Read the model definition and answer for the solid it produces. Units are mm, in the model's axes. A direction names the side the tool comes from. Give positions to 0.01 mm unless a question says otherwise; leave off trailing zeros. Order: outer loops, then holes, each group sorted by start corner. A loop starts at its lowest first (then second) coordinate and runs counter-clockwise, first axis right, second up. Notation, with made-up numbers: M 76,20 L 127,20 A22 ccw 127,36 Z; hole C 74.25,26 d5. An arc over 180 degrees is marked long. One line per item, written item: value.
from build123d import *

# Parameters (mm, degrees)
SKETCH2_W                       = 200
SKETCH2_H                       = 50
SKETCH2_R                       = 19
SKETCH2_R_2                     = 3.55
BOSS_EXTRUDE1_DEPTH             = 5
BOSS_EXTRUDE3_REACH             = 27
BOSS_EXTRUDE3_DIRECTION_2_REACH = 27
CUT_EXTRUDE2_DEPTH              = 20
CUT_EXTRUDE2_DEPTH_BACK         = 20
SKETCH8_R                       = 12.75
SKETCH8_R_2                     = 10.05
BOSS_EXTRUDE4_DEPTH             = 30.2
FILLET1_R                       = 5
SKETCH9_R                       = 3.5
CUT_EXTRUDE3_DEPTH              = 51
SKETCH13_R                      = 2
CUT_EXTRUDE5_DEPTH              = 2.5
CUT_EXTRUDE6_DEPTH              = 6
BOSS_EXTRUDE7_DEPTH             = 72
SKETCH17_R                      = 7.5
BOSS_EXTRUDE8_DEPTH             = 4
SKETCH18_R                      = 10.05
BOSS_EXTRUDE9_DEPTH             = 9.5
SKETCH19_W                      = 2.5
SKETCH19_H                      = 10
BOSS_EXTRUDE10_DEPTH            = 20
SKETCH20_R                      = 2.5
CUT_EXTRUDE7_DEPTH              = 36
SKETCH21_W                      = 3.5
SKETCH21_H                      = 5
CUT_EXTRUDE8_DEPTH              = 54.5


with BuildPart() as part:
    # Sketch2 → Boss-Extrude1 (new body)
    with BuildSketch(Plane(origin=(0, 0, 0), x_dir=(1, 0, 0), z_dir=(0, 1, 0))):
        Rectangle(SKETCH2_W, SKETCH2_H)
        with Locations((-60, 0)):
            Circle(SKETCH2_R, mode=Mode.SUBTRACT)
        with Locations((-31, 0)):
            Circle(SKETCH2_R_2, mode=Mode.SUBTRACT)
        with Locations((-89, 0)):
            Circle(SKETCH2_R_2, mode=Mode.SUBTRACT)
    extrude(amount=BOSS_EXTRUDE1_DEPTH)

    # Boss-Extrude3: up to this face of the body (flat: up to its plane)
    boss_extrude3_end = Plane(part.part.faces().sort_by_distance((0, 2.5, -25))[0])
    # Sketch6 → Boss-Extrude3 (add, up to the picked face)
    with BuildSketch(Plane.XY, mode=Mode.PRIVATE) as boss_extrude3_sk1:
        with BuildLine():
            Line((-100, 5), (-2.990738274, 34.75169137))
            ThreePointArc((-2.990738274, 34.75169137), (0, 35.2), (2.990738274, 34.75169137))
            Line((2.990738274, 34.75169137), (100, 5))
            Line((100, 5), (-100, 5))
        make_face()
    boss_extrude3_tool1 = split(extrude(boss_extrude3_sk1.sketch, amount=-BOSS_EXTRUDE3_REACH, mode=Mode.PRIVATE), bisect_by=boss_extrude3_end, keep=Keep.BOTH, mode=Mode.PRIVATE)
    add(boss_extrude3_tool1.solids().sort_by_distance((0, 15.216769, 0))[0])

    # Boss-Extrude3 direction 2: up to this face of the body (flat: up to its plane)
    boss_extrude3_direction_2_end = Plane(part.part.faces().sort_by_distance((0, 2.5, 25))[0])
    # Sketch6 → Boss-Extrude3 direction 2 (add, up to the picked face)
    with BuildSketch(Plane.XY, mode=Mode.PRIVATE) as boss_extrude3_direction_2_sk1:
        with BuildLine():
            Line((-100, 5), (-2.990738274, 34.75169137))
            ThreePointArc((-2.990738274, 34.75169137), (0, 35.2), (2.990738274, 34.75169137))
            Line((2.990738274, 34.75169137), (100, 5))
            Line((100, 5), (-100, 5))
        make_face()
    boss_extrude3_direction_2_tool1 = split(extrude(boss_extrude3_direction_2_sk1.sketch, amount=BOSS_EXTRUDE3_DIRECTION_2_REACH, mode=Mode.PRIVATE), bisect_by=boss_extrude3_direction_2_end, keep=Keep.BOTH, mode=Mode.PRIVATE)
    add(boss_extrude3_direction_2_tool1.solids().sort_by_distance((0, 15.216769, 0))[0])

    # Sketch7 → Cut-Extrude2 (cut, two sides)
    with BuildSketch(Plane.XY) as cut_extrude2_sk:
        with BuildLine():
            Line((2.990738274, 34.75169137), (100, 5))
            Line((100, 5), (-100, 5))
            Line((-100, 5), (-2.990738274, 34.75169137))
            ThreePointArc((-2.990738274, 34.75169137), (0, 35.2), (2.990738274, 34.75169137))
        make_face()
    extrude(amount=CUT_EXTRUDE2_DEPTH, mode=Mode.SUBTRACT)
    extrude(cut_extrude2_sk.sketch, amount=-CUT_EXTRUDE2_DEPTH_BACK, mode=Mode.SUBTRACT)

    # Sketch8 → Boss-Extrude4 (add)
    with BuildSketch(Plane(origin=(0, 5, 0), x_dir=(1, 0, 0), z_dir=(0, 1, 0))):
        Circle(SKETCH8_R)
        Circle(SKETCH8_R_2, mode=Mode.SUBTRACT)
    extrude(amount=BOSS_EXTRUDE4_DEPTH)

    # Fillet1
    fillet1_edges = [part.edges().sort_by_distance(p)[0] for p in [
        (0, 0, -25),
        (0, 0, 25),
    ]]
    fillet(fillet1_edges, radius=FILLET1_R)

    # Sketch9 → Cut-Extrude3 (cut, through all)
    with BuildSketch(Plane.XY.offset(25)):
        with Locations((0, 25)):
            Circle(SKETCH9_R)
    extrude(amount=-CUT_EXTRUDE3_DEPTH, mode=Mode.SUBTRACT)

    # Sketch13 → Cut-Extrude5 (cut)
    with BuildSketch(Plane(origin=(0, 5, 0), x_dir=(1, 0, 0), z_dir=(0, 1, 0))):
        with BuildLine():
            Line((23.5, 7.5), (53.5, 7.5))
            ThreePointArc((53.5, 7.5), (61, 0), (53.5, -7.5))
            Line((53.5, -7.5), (23.5, -7.5))
            ThreePointArc((23.5, -7.5), (16, 0), (23.5, 7.5))
        make_face()
        with Locations((31.5, 0)):
            Circle(SKETCH13_R, mode=Mode.SUBTRACT)
        with Locations((24.5, 0)):
            Circle(SKETCH13_R, mode=Mode.SUBTRACT)
        with Locations((38.5, 0)):
            Circle(SKETCH13_R, mode=Mode.SUBTRACT)
        with Locations((45.5, 0)):
            Circle(SKETCH13_R, mode=Mode.SUBTRACT)
        with Locations((52.5, 0)):
            Circle(SKETCH13_R, mode=Mode.SUBTRACT)
    extrude(amount=-CUT_EXTRUDE5_DEPTH, mode=Mode.SUBTRACT)

    # Sketch15 → Cut-Extrude6 (cut, through all)
    with BuildSketch(Plane(origin=(0, 5, 0), x_dir=(1, 0, 0), z_dir=(0, 1, 0))):
        with BuildLine():
            Line((23.5, 4), (53.5, 4))
            Line((53.5, 4), (100, 4))
            Line((100, 4), (100, -4))
            Line((100, -4), (53.5, -4))
            Line((53.5, -4), (23.5, -4))
            ThreePointArc((23.5, -4), (19.5, 0), (23.5, 4))
        make_face()
    extrude(amount=-CUT_EXTRUDE6_DEPTH, mode=Mode.SUBTRACT)

    # Sketch16 → Boss-Extrude7 (add)
    with BuildSketch(Plane(origin=(0, 5, 0), x_dir=(1, 0, 0), z_dir=(0, 1, 0))):
        with BuildLine():
            Line((16, -4), (16, -6.614378278))
            ThreePointArc((16, -6.614378278), (19.385621722, -9.114378278), (23.5, -10))
            Line((23.5, -10), (53.5, -10))
            Line((53.5, -10), (53.5, -7.5))
            Line((53.5, -7.5), (23.5, -7.5))
            ThreePointArc((23.5, -7.5), (19.877155813, -6.566962768), (17.15571123, -4))
            Line((17.15571123, -4), (16, -4))
        make_face()
        with BuildLine():
            Line((53.5, 10), (23.5, 10))
            ThreePointArc((23.5, 10), (19.385621722, 9.114378278), (16, 6.614378278))
            Line((16, 6.614378278), (16, 4))
            Line((16, 4), (17.15571123, 4))
            ThreePointArc((17.15571123, 4), (19.877155813, 6.566962768), (23.5, 7.5))
            Line((23.5, 7.5), (53.5, 7.5))
            Line((53.5, 7.5), (53.5, 10))
        make_face()
    extrude(amount=BOSS_EXTRUDE7_DEPTH)

    # Sketch17 → Boss-Extrude8 (add)
    with BuildSketch(Plane(origin=(0, 77, 0), x_dir=(1, 0, 0), z_dir=(0, 1, 0))):
        with BuildLine():
            Line((23.5, -10), (53.5, -10))
            Line((53.5, -10), (53.5, 10))
            Line((53.5, 10), (23.5, 10))
            ThreePointArc((23.5, 10), (19.385621722, 9.114378278), (16, 6.614378278))
            Line((16, 6.614378278), (16, 4))
            Line((16, 4), (16, -4))
            Line((16, -4), (16, -6.614378278))
            ThreePointArc((16, -6.614378278), (19.385621722, -9.114378278), (23.5, -10))
        make_face()
        with Locations((38.5, 0)):
            Circle(SKETCH17_R, mode=Mode.SUBTRACT)
    extrude(amount=BOSS_EXTRUDE8_DEPTH)

    # Sketch18 → Boss-Extrude9 (add)
    with BuildSketch(Plane(origin=(0, 5, 0), x_dir=(1, 0, 0), z_dir=(0, 1, 0))):
        Circle(SKETCH18_R)
    extrude(amount=BOSS_EXTRUDE9_DEPTH)

    # Sketch19 → Boss-Extrude10 (add)
    with BuildSketch(Plane(origin=(53.5, 0, 0), x_dir=(0, 0, -1), z_dir=(1, 0, 0))):
        with Locations((-8.75, 57)):
            Rectangle(SKETCH19_W, SKETCH19_H)
        with Locations((8.75, 57)):
            Rectangle(SKETCH19_W, SKETCH19_H)
        with Locations((8.75, 29)):
            Rectangle(SKETCH19_W, SKETCH19_H)
        with Locations((-8.75, 29)):
            Rectangle(SKETCH19_W, SKETCH19_H)
    extrude(amount=BOSS_EXTRUDE10_DEPTH)

    # Sketch20 → Cut-Extrude7 (cut, through all)
    with BuildSketch(Plane.XY.offset(10)):
        with Locations((66, 57)):
            Circle(SKETCH20_R)
        with Locations((66, 29)):
            Circle(SKETCH20_R)
    extrude(amount=-CUT_EXTRUDE7_DEPTH, mode=Mode.SUBTRACT)

    # Sketch21 → Cut-Extrude8 (cut)
    with BuildSketch(Plane(origin=(100, 0, 0), x_dir=(0, 0, -1), z_dir=(1, 0, 0))):
        with Locations((-5.75, 2.5)):
            Rectangle(SKETCH21_W, SKETCH21_H)
        with Locations((5.75, 2.5)):
            Rectangle(SKETCH21_W, SKETCH21_H)
    extrude(amount=-CUT_EXTRUDE8_DEPTH, mode=Mode.SUBTRACT)


solid = part.part
1) Consider probe 1 along Z at (x, y) = (36.5, 16); probe 2 along Y at (x, z) = (66, -8.2); probe 3 along Z at (x, y) = (-24.5, 6). Determine where each line is inside the solid, lowest interval first.
Reported:
probe 1: z = -25 to -20, -10 to -7.5, 7.5 to 10, 20 to 25
probe 2: y = 0 to 5, 24 to 26.5, 31.5 to 34, 52 to 54.5, 59.5 to 62
probe 3: z = -25 to -20, 20 to 25
2) Determine the mould class of faces 6 (the face through (1, 2, 24)), 7 (the face through (-1, 13, -25)), 8 (the face through (31, 2.5, 5)) for opening direction Y: +Y half, -Y half, draft (parallel to the pull), parting line (faces both ways), or undercut.
Reported:
face 6: -Y half
face 7: draft
face 8: undercut
3) Find section D-D, the plane x = 41. Write down the section's boundary in (y, z), plus the area to 3 significant figures.
Reported:
outline: M 0,-20 A5 ccw 5,-25 L 23.09,-25 L 23.09,-20 L 5,-20 L 5,-10 L 81,-10 L 81,-7.07 L 77,-7.07 L 77,-7.5 L 2.5,-7.5 L 2.5,-4 L 0,-4 Z; M 0,4 L 2.5,4 L 2.5,7.5 L 77,7.5 L 77,7.07 L 81,7.07 L 81,10 L 5,10 L 5,20 L 23.09,20 L 23.09,25 L 5,25 A5 ccw 0,20 Z
area: 746 mm^2
4) Find section C-C, the plane x = -56. Write down the section's boundary in (y, z).
Reported:
outline: M 0,-20 A5 ccw 5,-25 L 18.49,-25 L 18.49,-20 L 5,-20 L 5,-18.57 L 0,-18.57 Z; M 0,18.57 L 5,18.57 L 5,20 L 18.49,20 L 18.49,25 L 5,25 A5 ccw 0,20 Z
5) Which of the six approach directions +Z, -Z, +X, -X, +Y, -Y give full straight-line access (tool end or side, diameter ignored) to faces 1 (the face through (1, 14, -20)), 2 (the face through (43, 42, 10)), 3 (the face through (53.5, 78, 0)), 4 (the face through (45, 29, -7.5)), 5 (the face through (19.33, 42.47, 9.09))?
Reported:
face 1: +X, -X, +Y
face 2: +X, +Y
face 3: +Z, -Z, +X, +Y
face 4: +X
face 5: +Y
6) Find section B-B, the plane y = 75. Write down the section's boundary in (x, z).
Reported:
outline: M 16,-6.61 A10 ccw 23.5,-10 L 53.5,-10 L 53.5,-7.5 L 23.5,-7.5 A7.5 cw 17.16,-4 L 16,-4 Z; M 16,4 L 17.16,4 A7.5 cw 23.5,7.5 L 53.5,7.5 L 53.5,10 L 23.5,10 A10 ccw 16,6.61 Z
7) Find section A-A, the plane z = 0. Count the separate pieces of the cut face and the enclosed holes in it, plus the area to 3 significant figures.
Reported:
separate pieces: 6
enclosed holes: 0
area: 772 mm^2
8) Each of these flat-tipped pins is pushed along its axis until it touches: pin 1 Ø23 at (x, y) = (80.5, 45.5) entering from -Z; pin 2 Ø2 at (x, y) = (23, 49.5) entering from +Z; pin 3 Ø10.5 at (y, z) = (31, 2.5) entering from -X. Where does it stop, or does it pass through?
Reported:
pin 1: stops at z = -10
pin 2: stops at z = 10
pin 3: stops at x = -12.75
